Input: part model. Units: mm. Frame: model coordinates. A direction names the side the tool comes from. Coordinates: 2 decimals unless noted, no trailing zeros. Write each loop counter-clockwise with the first axis right and the second up, starting at its lowest first coordinate (ties: lowest second). Pieces come first, ordered by that corner, then holes. Notation, with made-up numbers: M -10.75,-32 L 42.25,-32 A25 ccw 42.25,0 Z; hole C 48,-20 d7. An arc over 180 degrees is marked long. Use one line per item in the form item = value.
from build123d import *

# Parameters (mm, degrees)
SKETCH1_W                     = 32
SKETCH1_H                     = 27.5
BOSS_EXTRUDE1_DEPTH           = 4
SKETCH2_W                     = 8
SKETCH2_H                     = 14.5
CUT_EXTRUDE1_DEPTH            = 42.112650121
SKETCH3_W                     = 16
SKETCH3_H                     = 6.5
CUT_EXTRUDE2_DEPTH            = 42.112650121
DRAFT1_ANGLE                  = 35.000000002
F_3_0_3_DIAMETER_HOLE1_D      = 3
CSK_FOR_M3_SFHCS1_D           = 2.2
CSK_FOR_M3_SFHCS1_DEPTH       = 9.5
CSK_FOR_M3_SFHCS1_CSINK_D     = 4.6
CSK_FOR_M3_SFHCS1_CSINK_ANGLE = 90
CSK_FOR_M3_SFHCS1_TIP         = 0.660946681
M3X0_5_TAPPED_HOLE2_D         = 2.5
M3X0_5_TAPPED_HOLE2_DEPTH     = 7.5
M3X0_5_TAPPED_HOLE2_TIP       = 0.751075774
FILLET1_R                     = 1
FILLET2_R                     = 2
FILLET3_R                     = 3
FILLET4_R                     = 4
M3X0_5_TAPPED_HOLE1_D         = 2.5


with BuildPart() as part:
    # Sketch1 → Boss-Extrude1 (new body)
    with BuildSketch(Plane.XY.offset(4)):
        with Locations((16, 11.75)):
            Rectangle(SKETCH1_W, SKETCH1_H)
    extrude(amount=-BOSS_EXTRUDE1_DEPTH)

    # Sketch2 → Cut-Extrude1 (cut, through all)
    with BuildSketch(Plane(origin=(0, 0, 0), x_dir=(-1, 0, 0), z_dir=(0, 0, -1))):
        with Locations((-4, 18.25)):
            Rectangle(SKETCH2_W, SKETCH2_H)
    extrude(amount=-CUT_EXTRUDE1_DEPTH, mode=Mode.SUBTRACT)

    # Sketch3 → Cut-Extrude2 (cut, through all)
    with BuildSketch(Plane(origin=(0, 0, 0), x_dir=(-1, 0, 0), z_dir=(0, 0, -1))):
        with Locations((-16, 22.25)):
            Rectangle(SKETCH3_W, SKETCH3_H)
    extrude(amount=-CUT_EXTRUDE2_DEPTH, mode=Mode.SUBTRACT)

    # Draft1
    draft1_faces = [part.faces().sort_by_distance(p)[0] for p in [
        (28, 25.5, 2),
    ]]
    draft(draft1_faces, Plane(origin=(24, 25.5, 4), x_dir=(0, 0, -1), z_dir=(-1, 0, 0)), DRAFT1_ANGLE)

    # Ø3.0 (3) Diameter Hole1 (through all)
    with Locations(Plane(origin=(0, 0, 0), x_dir=(-1, 0, 0), z_dir=(0, 0, -1))):
        with Locations((-27, 24)):
            Hole(F_3_0_3_DIAMETER_HOLE1_D / 2)

    # CSK for M3 SFHCS1
    with Locations(Plane(origin=(0, 0, 0), x_dir=(-1, 0, 0), z_dir=(0, 0, -1))):
        with Locations((-29.4, 27.2)):
            CounterSinkHole(CSK_FOR_M3_SFHCS1_D / 2, CSK_FOR_M3_SFHCS1_CSINK_D / 2, depth=CSK_FOR_M3_SFHCS1_DEPTH, counter_sink_angle=CSK_FOR_M3_SFHCS1_CSINK_ANGLE)
            with Locations((0, 0, -(CSK_FOR_M3_SFHCS1_DEPTH + CSK_FOR_M3_SFHCS1_TIP / 2))):  # 118° drill point
                Cone(0, CSK_FOR_M3_SFHCS1_D / 2, CSK_FOR_M3_SFHCS1_TIP, mode=Mode.SUBTRACT)

    # M3x0.5 Tapped Hole2
    with Locations(Plane(origin=(0, -2, 0), x_dir=(-1, 0, 0), z_dir=(0, -1, 0))):
        with Locations((-10, -2), (-19.5, -2), (-29, -2)):
            Hole(M3X0_5_TAPPED_HOLE2_D / 2, depth=M3X0_5_TAPPED_HOLE2_DEPTH)
            with Locations((0, 0, -(M3X0_5_TAPPED_HOLE2_DEPTH + M3X0_5_TAPPED_HOLE2_TIP / 2))):  # 118° drill point
                Cone(0, M3X0_5_TAPPED_HOLE2_D / 2, M3X0_5_TAPPED_HOLE2_TIP, mode=Mode.SUBTRACT)

    # Fillet1
    fillet1_edges = [part.edges().sort_by_distance(p)[0] for p in [
        (8, 11, 2),
    ]]
    fillet(fillet1_edges, radius=FILLET1_R)

    # Fillet2
    fillet2_edges = [part.edges().sort_by_distance(p)[0] for p in [
        (24, 19, 2),
    ]]
    fillet(fillet2_edges, radius=FILLET2_R)

    # Fillet3
    fillet3_edges = [part.edges().sort_by_distance(p)[0] for p in [
        (0, 11, 2),
    ]]
    fillet(fillet3_edges, radius=FILLET3_R)

    # Fillet4
    fillet4_edges = [part.edges().sort_by_distance(p)[0] for p in [
        (8, 19, 2),
    ]]
    fillet(fillet4_edges, radius=FILLET4_R)

    # M3x0.5 Tapped Hole1 (through all)
    with Locations(Plane(origin=(6, 5, 0), x_dir=(-1, 0, 0), z_dir=(0, 0, -1))):
        with Locations((0, 0)):
            Hole(M3X0_5_TAPPED_HOLE1_D / 2)


solid = part.part
(1) Section query C-C on x = 24.5. Return the cut outline in (y, z), plus the area to 3 significant figures.
Computed:
outline = M -2,0 L 25.85,0 L 25.85,4 L -2,4 Z
area = 111 mm^2
(2) Section query B-B on y = 13.5. Return the cut outline in (x, z), plus the area to 3 significant figures.
Computed:
outline = M 8,0 L 32,0 L 32,4 L 8,4 Z
area = 96.0 mm^2
(3) Set-up query: faces 1 (the cylindrical face through (30.19, 1.8, 1.62)), 2 (the flat face through (8, 13, 2)), 3 (the flat face through (19, 11, 4)). Return all of +Z, -Z, +X, -X, +Y, -Y with unobstructed straight access to the full face (end or side cutting, diameter ignored); none if empty.
Computed:
face_1 = -Y
face_2 = +Z, -Z, -X, +Y
face_3 = +Z, +X, -X, +Y, -Y
(4) Line query: probe 1 along X at (y, z) = (2, 2.6); probe 2 along Y at (x, z) = (27, 1.2); probe 3 along Y at (x, z) = (31, 0.2). Output: solid intervals per line, ascending.
Computed:
probe_1 = 0 to 8.9, 11.1 to 18.4, 20.6 to 27.9, 30.1 to 32
probe_2 = -2 to 22.5, 25.5 to 27.6
probe_3 = -2 to 25.84, 28.56 to 30.4
(5) Section query A-A on y = 24. Return the cut outline in (x, z), plus the area to 3 significant figures.
Computed:
outline = M 24,0 L 25.5,0 L 25.5,4 L 24,4 Z; M 28.5,0 L 32,0 L 32,4 L 28.5,4 Z
area = 20.0 mm^2
(6) First-contact query: pin 1 Ø3 at (x, y) = (26, 9.5) entering from -Z; pin 2 Ø2 at (x, y) = (6, 5) entering from -Z; pin 3 Ø1 at (x, z) = (10, 3) entering from +Y; pin 4 Ø1 at (y, z) = (15.5, 2) entering from -X. Flat tips, straight axial feed; report the tip coordinate or a pass-through.
Computed:
pin_1 = 0
pin_2 = through
pin_3 = 18.71
pin_4 = 8
(7) Pull-direction query (Y, two-part tool) for faces 4 (the conical face through (29.996, 26.054, 1.008)), 5 (the cylindrical face through (23.4, 19.57, 2.03)), 6 (the flat face through (16, -2, 2)); classes: pulls with the +Y half, pulls with the -Y half, needs draft (parallel to the pull), parting line crosses it, or undercut.
Computed:
face_4 = undercut
face_5 = pulls with the +Y half
face_6 = pulls with the -Y half
